```python
from build123d import *

# Parameters (mm, degrees)
BOX_W                   = 10
BOX_H                   = 10
BOX_DEPTH               = 10
EXTRUDE_DEPTH           = 125
LINK001_PLACEMENT_ANGLE = 270


with BuildPart() as cube:
    # Box → Box (new body)
    with BuildSketch(Plane(origin=(-52.5, -10, -18.8), x_dir=(1, 0, 0), z_dir=(0, 0, 1))):
        with Locations((5, 5)):
            Rectangle(BOX_W, BOX_H)
    extrude(amount=BOX_DEPTH)


with BuildPart() as cut:
    # Sketch001 → Extrude (new body)
    with BuildSketch(Plane.XZ):
        Polygon((-60.5, 0), (-60.5, -0.3), (-57.5, -0.3), (-57.5, -13.8), (-52.5, -13.8), (-52.5, -18.8), (-62.5, -18.8), (-62.5, 0), align=None)
    extrude(amount=EXTRUDE_DEPTH)


with BuildPart() as cut_1:
    # Link001 placement: moved
    add(cut.part.moved(Location((62.5, -62.5, 0))).rotate(Axis((62.5, -62.5, 0), (0, 0, 1)), LINK001_PLACEMENT_ANGLE))

    # Cut: cut Cube
    add(cube.part, mode=Mode.SUBTRACT)


solid = cut_1.part
```
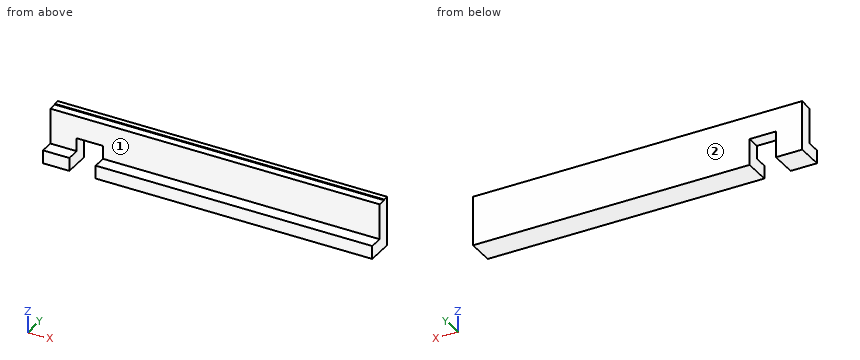
Can you work these out from the model? Positions are in its coordinate system, mm. Face numbers are marked on the shaded views. A direction names the side the tool comes from. Give positions to 0.01 mm unless a question says otherwise; leave off trailing zeros. Loops run counter-clockwise (first coordinate to the right, second up) from the corner with the lowest first, then second, coordinate; pieces in that order, holes last. Notation, with made-up numbers: M 80.25,-38.5 L 93.25,-38.5 A20 ccw 93.25,-13.5 Z; hole C -8.5,1 d1. An arc over 180 degrees is marked long. Use CSV: the item, a comma, the result in double quotes. Start each with the question number.
1. If I drill on L1, parallel to X at y = -2.25, z = -16.75; L2, parallel to Z at x = 13, y = -9; L3, parallel to Z at x = 43, y = -2.5, over which ranges is the centre line in solid material (lowest first)?
2. On a 3-axis mill with a long thin cutter (end or side, diameter ignored), from which of +Z, -Z, +X, -X, +Y, -Y can I reach the whole of each face in a straight line? I mean the marked faces 1 and 2. Say none if no direction works.
3. Imagine slicing it at B-B, the plane z = -12. Write out the boundary of the cut face in (x, y).
4. Imagine slicing it at D-D, the plane z = -6.5. Write out the boundary of the cut face in (x, y).
5. Imagine slicing it at A-A, the plane y = -8. Write out the boundary of the cut face in (x, z), plus the area to 3 significant figures.
6. Imagine slicing it at C-C, the plane x = 48.5. Write out the boundary of the cut face in (y, z), plus the area to 3 significant figures.
7. For P1, Ø2.5, axis at x = -45.5, y = -3, coming from the -Z side; P2, Ø6, axis at x = -37, y = -5.5, coming from the +Z side; P3, Ø1.5, axis at x = -57.5, y = -6.5, coming from the +Z side, each with a flat end and sliding along its axis, tell me the tip position at first contact or that it passes through.
Response values:
1,L1,"-62.5 to -52.5, -42.5 to 62.5"
1,L2,"-18.8 to -13.8"
1,L3,"-18.8 to -0.3"
2,face 1,"+Z, +X, -X, -Y"
2,face 2,"+Z, -Z, +X, -X, +Y"
3,outline,"M -62.5,-5 L -52.5,-5 L -52.5,0 L -62.5,0 Z; M -42.5,-5 L 62.5,-5 L 62.5,0 L -42.5,0 Z"
4,outline,"M -62.5,-5 L 62.5,-5 L 62.5,0 L -62.5,0 Z"
5,outline,"M -62.5,-18.8 L -52.5,-18.8 L -52.5,-13.8 L -62.5,-13.8 Z; M -42.5,-18.8 L 62.5,-18.8 L 62.5,-13.8 L -42.5,-13.8 Z"
5,area,"575 mm^2"
6,outline,"M -10,-18.8 L 0,-18.8 L 0,0 L -2,0 L -2,-0.3 L -5,-0.3 L -5,-13.8 L -10,-13.8 Z"
6,area,"118 mm^2"
7,P1,"z = -8.8"
7,P2,"z = -0.3"
7,P3,"z = -13.8"
